Design review of the part shown in the three views and the two pictorial views. Dimensions are in mm from the part's minimum x, y and z. Coordinates: 2 decimals unless noted, no trailing zeros. Write each loop counter-clockwise with the first axis right and the second up, starting at its lowest first coordinate (ties: lowest second). Pieces come first, ordered by that corner, then holes. Notation, with made-up numbers: (50.5, 61) -> (59.5, 61) arc R21 ccw to (59.5, 94) -> close; hole circle Ø10 at (-24, 69). An arc over 180 degrees is marked (long way). Write item = value, one per line. Start each with the question number.
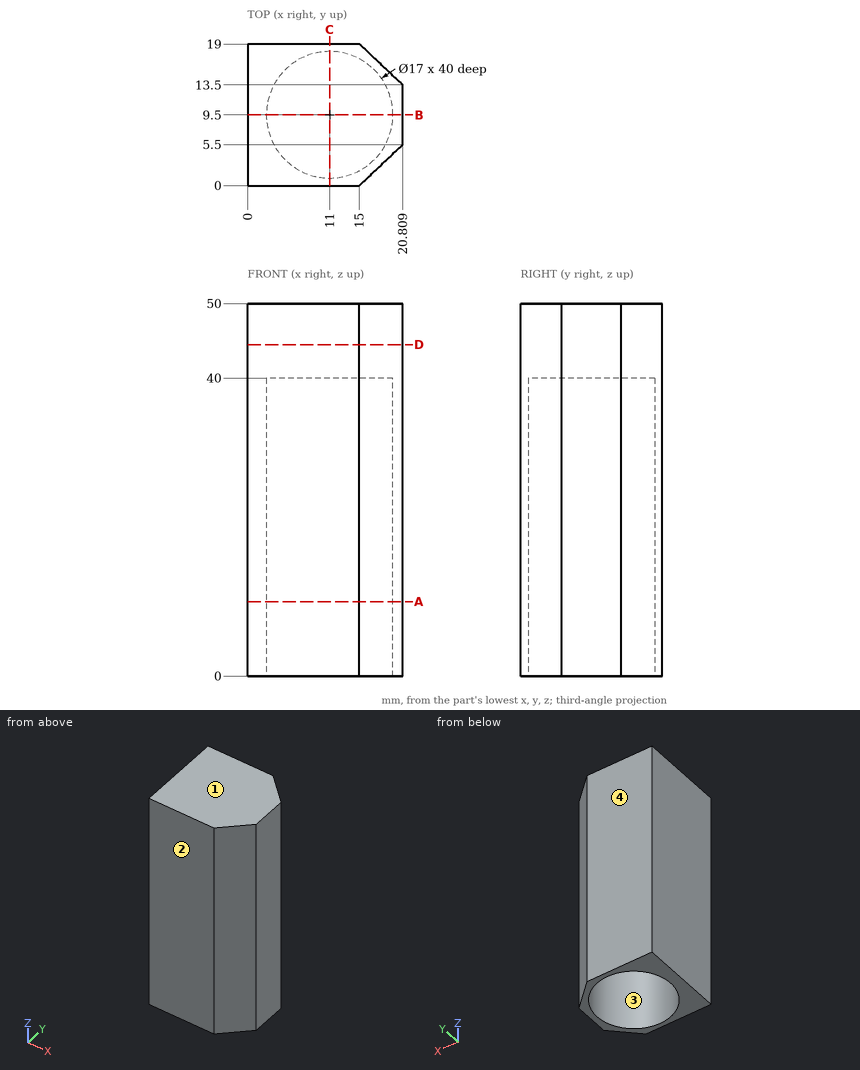
(1) Take a section at B-B, the plane y = 9.5. State the section outline as (x, z) points.
(2) Mouldability with a two-part tool opening along Y and no side actions: class the marked faces 1, 2, 3 and 4 as pulls with the +Y half, pulls with the -Y half, needs draft (parallel to the pull), parting line crosses it, or undercut.
(3) For pin 1 Ø1.5 at (y, z) = (3, 43.5) entering from +X; pin 2 Ø6 at (y, z) = (4.5, 8) entering from +X; pin 3 Ø5 at (x, y) = (9.5, 15) entering from -Z, all flat-tipped, find the tip position at first contact; note any pin that passes through.
(4) Take a section at C-C, the plane x = 11. State the section outline as (y, z) points, then the cut area to 3 significant figures.
(5) Take a section at A-A, the plane z = 10. State the section outline as (x, y) points.
(6) For line 1 (Y direction, x = 11, z = 19.5); line 2 (Z direction, x = 11, y = 10.5); line 3 (X direction, y = 14.75, z = 20) (1 decimal), list the stretches that pass through material, from the lowest coordinate up.
(7) Take a section at D-D, the plane z = 44.5. State the section outline as (x, y) points.
Report:
q1.outline = (0, 0) -> (2.5, 0) -> (2.5, 40) -> (19.5, 40) -> (19.5, 0) -> (20.81, 0) -> (20.81, 50) -> (0, 50) -> close
q2.face_1 = needs draft
q2.face_2 = pulls with the -Y half
q2.face_3 = undercut
q2.face_4 = pulls with the +Y half
q3.pin_1 = 18.96
q3.pin_2 = 20.81
q3.pin_3 = 40
q4.outline = (0, 0) -> (1, 0) -> (1, 40) -> (18, 40) -> (18, 0) -> (19, 0) -> (19, 50) -> (0, 50) -> close
q4.area = 270 mm2
q5.outline = (0, 0) -> (15, 0) -> (20.81, 5.5) -> (20.81, 13.5) -> (15, 19) -> (0, 19) -> close; hole circle Ø17 at (11, 9.5)
q6.line_1 = 0 to 1, 18 to 19
q6.line_2 = 40 to 50
q6.line_3 = 0 to 4.3, 17.7 to 19.5
q7.outline = (0, 0) -> (15, 0) -> (20.81, 5.5) -> (20.81, 13.5) -> (15, 19) -> (0, 19) -> close
